```python
from build123d import *

# Parameters (mm, degrees)
BOSS_EXTRUDE1_DEPTH = 80
SHELL1_T            = -3
SKETCH3_W           = 46
SKETCH3_H           = 47
BOSS_EXTRUDE2_DEPTH = 17
SKETCH4_W           = 10.2
SKETCH4_H           = 10.2
CUT_EXTRUDE1_DEPTH  = 20
SKETCH6_W           = 15
SKETCH6_H           = 12.8
CUT_EXTRUDE2_DEPTH  = 3
SKETCH7_W           = 40.4
SKETCH7_H           = 50
CUT_EXTRUDE3_DEPTH  = 5
FILLET1_R           = 4
CUT_EXTRUDE7_DEPTH  = 47
SKETCH13_R          = 1.5
CUT_EXTRUDE8_DEPTH  = 25
SKETCH14_R          = 3.1
CUT_EXTRUDE9_DEPTH  = 2
SKETCH17_W          = 45
SKETCH17_H          = 5
BOSS_EXTRUDE5_DEPTH = 74
CUT_EXTRUDE10_REACH = 48.51
SKETCH18_W          = 54
SKETCH18_H          = 45
CUT_EXTRUDE11_REACH = 48.51
SKETCH19_R          = 1.45
BOSS_EXTRUDE6_DEPTH = 47
SKETCH22_R          = 1.45
CUT_EXTRUDE12_DEPTH = 70.509632224
CUT_EXTRUDE13_REACH = 82
SKETCH24_R          = 3.7
SKETCH24_W          = 2
SKETCH24_H          = 3
BOSS_EXTRUDE7_DEPTH = 74
SKETCH27_R          = 1.65
CUT_EXTRUDE14_DEPTH = 10
CUT_EXTRUDE15_START = -3
CUT_EXTRUDE15_DEPTH = 32
CUT_EXTRUDE16_DEPTH = 30
BOSS_EXTRUDE8_DEPTH = 20
SKETCH31_R          = 1.5
CUT_EXTRUDE17_DEPTH = 43.509632224
CUT_EXTRUDE18_DEPTH = 15
CUT_EXTRUDE19_REACH = 48.51
SKETCH33_W          = 10
SKETCH33_H          = 5
SKETCH34_R          = 1.6
CUT_EXTRUDE20_DEPTH = 70.509632224
CUT_EXTRUDE22_DEPTH = 14


with BuildPart() as part:
    # Sketch2 → Boss-Extrude1 (new body)
    with BuildSketch(Plane(origin=(0, 0, 0), x_dir=(0, 0, -1), z_dir=(1, 0, 0))):
        Polygon((-27.320490368, 20.998248687), (-27.320490368, -29.001751313), (12.679509632, -29.001751313), (12.679509632, -48.511383538), (27.679509632, -48.511383538), (82.679509632, 0.998248687), (82.679509632, 20.998248687), align=None)
    extrude(amount=BOSS_EXTRUDE1_DEPTH)

    # Shell1
    shell1_openings = [part.faces().sort_by_distance(p)[0] for p in [
        (40, 20.998248687, -27.679509632),
    ]]
    offset(amount=SHELL1_T, openings=shell1_openings, kind=Kind.INTERSECTION)

    # Sketch3 → Boss-Extrude2 (add)
    with BuildSketch(Plane(origin=(0, 0, 24.320490368), x_dir=(-1, 0, 0), z_dir=(0, 0, -1))):
        with Locations((-40, -2.501751313)):
            Rectangle(SKETCH3_W, SKETCH3_H)
    extrude(amount=BOSS_EXTRUDE2_DEPTH)

    # Sketch4 → Cut-Extrude1 (cut)
    with BuildSketch(Plane.XY.offset(27.320490368)):
        with Locations((40, -4.001751313)):
            Rectangle(SKETCH4_W, SKETCH4_H)
    extrude(amount=-CUT_EXTRUDE1_DEPTH, mode=Mode.SUBTRACT)

    # Sketch6 → Cut-Extrude2 (cut)
    with BuildSketch(Plane.XZ.offset(29.001751313)):
        with Locations((51.5, 0.920490368)):
            Rectangle(SKETCH6_W, SKETCH6_H)
        with Locations((28.5, 0.920490368)):
            Rectangle(SKETCH6_W, SKETCH6_H)
    extrude(amount=-CUT_EXTRUDE2_DEPTH, mode=Mode.SUBTRACT)

    # Sketch7 → Cut-Extrude3 (cut)
    with BuildSketch(Plane.XY.offset(27.320490368)):
        with Locations((40, -4.001751313)):
            Rectangle(SKETCH7_W, SKETCH7_H)
    extrude(amount=-CUT_EXTRUDE3_DEPTH, mode=Mode.SUBTRACT)

    # Fillet1
    fillet1_edges = [part.edges().sort_by_distance(p)[0] for p in [
        (19.8, -4.001751313, 27.320490368),
        (60.2, -4.001751313, 27.320490368),
        (80, -4.001751313, 27.320490368),
        (0, -4.001751313, 27.320490368),
    ]]
    fillet(fillet1_edges, radius=FILLET1_R)

    # Sketch12 → Cut-Extrude7 (cut)
    with BuildSketch(Plane(origin=(0, 20.998248687, 0), x_dir=(1, 0, 0), z_dir=(0, 1, 0))):
        Polygon((33, -7.320490368), (19.8, -12.320490368), (17, -24.320490368), (17, -7.320490368), align=None)
        Polygon((47, -7.320490368), (63, -7.320490368), (63, -24.320490368), (60.2, -12.320490368), align=None)
    extrude(amount=-CUT_EXTRUDE7_DEPTH, mode=Mode.SUBTRACT)

    # Sketch13 → Cut-Extrude8 (cut)
    with BuildSketch(Plane(origin=(0, 20.998248687, 0), x_dir=(1, 0, 0), z_dir=(0, 1, 0))):
        with Locations((26, -17.320490368)):
            Circle(SKETCH13_R)
        with Locations((54, -17.320490368)):
            Circle(SKETCH13_R)
    extrude(amount=-CUT_EXTRUDE8_DEPTH, mode=Mode.SUBTRACT)

    # Sketch14 → Cut-Extrude9 (cut)
    with BuildSketch(Plane(origin=(0, 20.998248687, 0), x_dir=(1, 0, 0), z_dir=(0, 1, 0))):
        with Locations((26, -17.320490368)):
            Circle(SKETCH14_R)
        with Locations((54, -17.320490368)):
            Circle(SKETCH14_R)
    extrude(amount=-CUT_EXTRUDE9_DEPTH, mode=Mode.SUBTRACT)

    # Sketch17 → Boss-Extrude5 (add)
    with BuildSketch(Plane.ZY.offset(-77)):
        with Locations((-23.179509632, -4.501751313)):
            Rectangle(SKETCH17_W, SKETCH17_H)
    extrude(amount=BOSS_EXTRUDE5_DEPTH)

    # Sketch18 → Cut-Extrude10 (cut, up to next)
    with BuildSketch(Plane(origin=(0, -2.001751313, 0), x_dir=(1, 0, 0), z_dir=(0, 1, 0)), mode=Mode.PRIVATE) as cut_extrude10_sk1:
        with Locations((40, 23.179509632)):
            Rectangle(SKETCH18_W, SKETCH18_H)
    cut_extrude10_tool1 = extrude(cut_extrude10_sk1.sketch, amount=-CUT_EXTRUDE10_REACH, mode=Mode.PRIVATE) & part.part
    add(cut_extrude10_tool1.solids().sort_by_distance((40, -2.001751, -23.17951))[0], mode=Mode.SUBTRACT)

    # Sketch19 → Cut-Extrude11 (cut, up to next)
    with BuildSketch(Plane(origin=(0, -2.001751313, 0), x_dir=(1, 0, 0), z_dir=(0, 1, 0)), mode=Mode.PRIVATE) as cut_extrude11_sk1:
        with Locations((72, 37.179509632)):
            Circle(SKETCH19_R)
    cut_extrude11_tool1 = extrude(cut_extrude11_sk1.sketch, amount=-CUT_EXTRUDE11_REACH, mode=Mode.PRIVATE) & part.part
    add(cut_extrude11_tool1.solids().sort_by_distance((72, -2.001751, -37.17951))[0], mode=Mode.SUBTRACT)
    # Sketch19 → Cut-Extrude11 (cut, up to next)
    with BuildSketch(Plane(origin=(0, -2.001751313, 0), x_dir=(1, 0, 0), z_dir=(0, 1, 0)), mode=Mode.PRIVATE) as cut_extrude11_sk2:
        with Locations((72, 6.179509632)):
            Circle(SKETCH19_R)
    cut_extrude11_tool2 = extrude(cut_extrude11_sk2.sketch, amount=-CUT_EXTRUDE11_REACH, mode=Mode.PRIVATE) & part.part
    add(cut_extrude11_tool2.solids().sort_by_distance((72, -2.001751, -6.17951))[0], mode=Mode.SUBTRACT)
    # Sketch19 → Cut-Extrude11 (cut, up to next)
    with BuildSketch(Plane(origin=(0, -2.001751313, 0), x_dir=(1, 0, 0), z_dir=(0, 1, 0)), mode=Mode.PRIVATE) as cut_extrude11_sk3:
        with Locations((8, 33.179509632)):
            Circle(SKETCH19_R)
    cut_extrude11_tool3 = extrude(cut_extrude11_sk3.sketch, amount=-CUT_EXTRUDE11_REACH, mode=Mode.PRIVATE) & part.part
    add(cut_extrude11_tool3.solids().sort_by_distance((8, -2.001751, -33.17951))[0], mode=Mode.SUBTRACT)
    # Sketch19 → Cut-Extrude11 (cut, up to next)
    with BuildSketch(Plane(origin=(0, -2.001751313, 0), x_dir=(1, 0, 0), z_dir=(0, 1, 0)), mode=Mode.PRIVATE) as cut_extrude11_sk4:
        with Locations((8, 6.179509632)):
            Circle(SKETCH19_R)
    cut_extrude11_tool4 = extrude(cut_extrude11_sk4.sketch, amount=-CUT_EXTRUDE11_REACH, mode=Mode.PRIVATE) & part.part
    add(cut_extrude11_tool4.solids().sort_by_distance((8, -2.001751, -6.17951))[0], mode=Mode.SUBTRACT)

    # Sketch21 → Boss-Extrude6 (add)
    with BuildSketch(Plane(origin=(0, -26.001751313, 0), x_dir=(1, 0, 0), z_dir=(0, 1, 0))):
        Polygon((3, -24.320490368), (3, -14.320490368), (19.333333333, -14.320490368), (17, -24.320490368), align=None)
    extrude(amount=BOSS_EXTRUDE6_DEPTH)

    # Sketch22 → Cut-Extrude12 (cut, through all)
    with BuildSketch(Plane(origin=(0, 20.998248687, 0), x_dir=(1, 0, 0), z_dir=(0, 1, 0))):
        with Locations((10, -19.320490368)):
            Circle(SKETCH22_R)
    extrude(amount=-CUT_EXTRUDE12_DEPTH, mode=Mode.SUBTRACT)

    # Sketch24 → Cut-Extrude13 (cut, up to next)
    with BuildSketch(Plane(origin=(80, 0, 0), x_dir=(0, 0, -1), z_dir=(1, 0, 0)), mode=Mode.PRIVATE) as cut_extrude13_sk1:
        with Locations((26.679509632, -30.511383538)):
            Circle(SKETCH24_R)
    cut_extrude13_tool1 = extrude(cut_extrude13_sk1.sketch, amount=-CUT_EXTRUDE13_REACH, mode=Mode.PRIVATE) & part.part
    add(cut_extrude13_tool1.solids().sort_by_distance((80, -30.511384, -26.67951))[0], mode=Mode.SUBTRACT)
    # Sketch24 → Cut-Extrude13 (cut, up to next)
    with BuildSketch(Plane(origin=(80, 0, 0), x_dir=(0, 0, -1), z_dir=(1, 0, 0)), mode=Mode.PRIVATE) as cut_extrude13_sk2:
        with Locations((34.379509632, -30.511383538)):
            Rectangle(SKETCH24_W, SKETCH24_H)
    cut_extrude13_tool2 = extrude(cut_extrude13_sk2.sketch, amount=-CUT_EXTRUDE13_REACH, mode=Mode.PRIVATE) & part.part
    add(cut_extrude13_tool2.solids().sort_by_distance((80, -30.511384, -34.37951))[0], mode=Mode.SUBTRACT)

    # Sketch26 → Boss-Extrude7 (add)
    with BuildSketch(Plane(origin=(3, 0, 0), x_dir=(0, 0, -1), z_dir=(1, 0, 0))):
        Polygon((79.679509632, 2.334161996), (63.679509632, 2.334161996), (63.679509632, -12.068640106), align=None)
    extrude(amount=BOSS_EXTRUDE7_DEPTH)

    # Sketch27 → Cut-Extrude14 (cut)
    with BuildSketch(Plane(origin=(0, 2.334161996, 0), x_dir=(1, 0, 0), z_dir=(0, 1, 0))):
        with Locations((6, 76.679509632)):
            Circle(SKETCH27_R)
        with Locations((74, 76.679509632)):
            Circle(SKETCH27_R)
    extrude(amount=-CUT_EXTRUDE14_DEPTH, mode=Mode.SUBTRACT)

    # Sketch28 → Cut-Extrude15 (cut)
    with BuildSketch(Plane(origin=(0, 2.334161996, 0), x_dir=(1, 0, 0), z_dir=(0, 1, 0)).offset(CUT_EXTRUDE15_START)):
        Polygon((74, 79.929509632), (71.185417438, 78.304509632), (71.185417438, 75.054509632), (74, 73.429509632), (76.814582562, 75.054509632), (76.814582562, 78.304509632), align=None)
        Polygon((6, 73.429509632), (8.814582562, 75.054509632), (8.814582562, 78.304509632), (6, 79.929509632), (3.185417438, 78.304509632), (3.185417438, 75.054509632), align=None)
    extrude(amount=-CUT_EXTRUDE15_DEPTH, mode=Mode.SUBTRACT)

    # Sketch29 → Cut-Extrude16 (cut)
    with BuildSketch(Plane.XZ.offset(29.001751313)):
        Polygon((7.185417438, 17.695490368), (10, 16.070490368), (12.814582562, 17.695490368), (12.814582562, 20.945490368), (10, 22.570490368), (7.185417438, 20.945490368), align=None)
    extrude(amount=-CUT_EXTRUDE16_DEPTH, mode=Mode.SUBTRACT)

    # Sketch30 → Boss-Extrude8 (add)
    with BuildSketch(Plane(origin=(0, -26.001751313, 0), x_dir=(1, 0, 0), z_dir=(0, 1, 0))):
        Polygon((77, -24.320490368), (63, -24.320490368), (60.2, -12.320490368), (77, -12.320490368), align=None)
    extrude(amount=BOSS_EXTRUDE8_DEPTH)

    # Sketch31 → Cut-Extrude17 (cut, through all)
    with BuildSketch(Plane(origin=(0, -6.001751313, 0), x_dir=(1, 0, 0), z_dir=(0, 1, 0))):
        with Locations((72, -21.320490368)):
            Circle(SKETCH31_R)
    extrude(amount=-CUT_EXTRUDE17_DEPTH, mode=Mode.SUBTRACT)

    # Sketch32 → Cut-Extrude18 (cut)
    with BuildSketch(Plane.XZ.offset(29.001751313)):
        Polygon((72, 24.570490368), (69.185417438, 22.945490368), (69.185417438, 19.695490368), (72, 18.070490368), (74.814582562, 19.695490368), (74.814582562, 22.945490368), align=None)
    extrude(amount=-CUT_EXTRUDE18_DEPTH, mode=Mode.SUBTRACT)

    # Sketch33 → Cut-Extrude19 (cut, up to next)
    with BuildSketch(Plane(origin=(0, -2.001751313, 0), x_dir=(1, 0, 0), z_dir=(0, 1, 0)), mode=Mode.PRIVATE) as cut_extrude19_sk1:
        with Locations((72, 43.179509632)):
            Rectangle(SKETCH33_W, SKETCH33_H)
    cut_extrude19_tool1 = extrude(cut_extrude19_sk1.sketch, amount=-CUT_EXTRUDE19_REACH, mode=Mode.PRIVATE) & part.part
    add(cut_extrude19_tool1.solids().sort_by_distance((72, -2.001751, -43.17951))[0], mode=Mode.SUBTRACT)

    # Sketch34 → Cut-Extrude20 (cut, through all)
    with BuildSketch(Plane(origin=(0, 20.998248687, 0), x_dir=(1, 0, 0), z_dir=(0, 1, 0))):
        with Locations((40, -17.320490368)):
            Circle(SKETCH34_R)
    extrude(amount=-CUT_EXTRUDE20_DEPTH, mode=Mode.SUBTRACT)

    # Sketch36 → Cut-Extrude22 (cut)
    with BuildSketch(Plane.XZ.offset(29.001751313)):
        Polygon((38.375, 20.13507293), (36.75, 17.320490368), (38.375, 14.505907805), (41.625, 14.505907805), (43.25, 17.320490368), (41.625, 20.13507293), align=None)
    extrude(amount=-CUT_EXTRUDE22_DEPTH, mode=Mode.SUBTRACT)


solid = part.part
```
Can you work these out from the model? Positions are in its coordinate system, mm. A direction names the side the tool comes from. Coordinates: 2 decimals unless noted, no trailing zeros. Loops run counter-clockwise (first coordinate to the right, second up) from the corner with the lowest first, then second, coordinate; pieces in that order, holes last. Notation, with made-up numbers: (57.5, 36.25) -> (79.5, 36.25) arc R28 cw to (79.5, 64.25) -> close; hole circle Ø1 at (13, 68). An arc over 180 degrees is marked (long way). Answer as a JSON object with one key per item and string values.
1) Imagine slicing it at C-C (x = 17.5). Please give me the cut outline in (y, z), then the cut area to 3 significant figures.
Results:
{"outline": "(-48.51, -27.68) -> (1, -82.68) -> (21, -82.68) -> (21, -79.68) -> (2.33, -79.68) -> (2.33, -63.68) -> (-12.07, -63.68) -> (-45.51, -26.53) -> (-45.51, -15.68) -> (-26, -15.68) -> (-26, 14.32) -> (21, 14.32) -> (21, 26.94) -> (-29, 26.94) -> (-29, -12.68) -> (-48.51, -12.68) -> close", "area": "1,210 mm^2"}
2) For faces 4 (the face through (73.388, -21.607, 18.872)), 5 (the face through (39, 12, -79.68)), 6 (the face through (36, -28, 1)), 7 (the face through (61.403, -3.652, 26.18)), 8 (the face through (78.521, -30.349, -22.983)), which set-ups out of +Z, -Z, +X, -X, +Y, -Y let a thin tool reach every point of the face, with its end or its side?
Results:
{"face 4": "-Y", "face 5": "+Y", "face 6": "+Y, -Y", "face 7": "+Z, +Y, -Y", "face 8": "+X"}
3) Thinking about a two-plate mould opening in X: for faces 1 (the face through (0, -6, -29)), 2 (the face through (7.185, -14, 19)), 3 (the face through (39, -48.511, -20)), which applies, pulls with the +X half, pulls with the -X half, needs draft (parallel to the pull), parting line crosses it, or undercut?
Results:
{"face 1": "pulls with the -X half", "face 2": "undercut", "face 3": "needs draft"}
4) Imagine slicing it at D-D (y = -23). Count the separate pieces of the cut face and the enclosed holes in it, then the cut area to 3 significant figures.
Results:
{"separate pieces": "1", "enclosed holes": "4", "area": "1,750 mm^2"}
5) If I drill on line 1 (Z direction, x = 74, y = 1); line 2 (X direction, y = -28, z = -0.5); line 3 (Z direction, x = 54, y = 20.5), over which ranges is the centre line in solid material (lowest first)?
Results:
{"line 1": "z = -82.68 to -78.33, -75.03 to -63.68, 24.32 to 27.32", "line 2": "x = 0 to 21, 36 to 44, 59 to 80", "line 3": "z = -82.68 to -79.68, 9.97 to 14.22, 20.42 to 22.32"}
6) For P1, Ø1, axis at x = 36.5, z = 1, coming from the -Y side; P2, Ø2.5, axis at x = 31, y = -27, coming from the +Z side; P3, Ø2.5, axis at x = 8, z = -33.18, coming from the -Y side, each with a flat end and sliding along its axis, tell me the tip position at first contact or that it passes through.
Results:
{"P1": "stops at y = -29", "P2": "stops at z = 22.32", "P3": "stops at y = -44.69"}
7) Imagine slicing it at A-A (y = 6.5). Please give me the cut outline in (x, z), then the cut area to 3 significant figures.
Results:
{"outline": "(0, -82.68) -> (80, -82.68) -> (80, 23.32) arc R4 ccw to (76, 27.32) -> (64.2, 27.32) arc R4 ccw to (60.2, 23.32) -> (60.2, 22.32) -> (19.8, 22.32) -> (19.8, 23.32) arc R4 ccw to (15.8, 27.32) -> (4, 27.32) arc R4 ccw to (0, 23.32) -> close; hole (3, -79.68) -> (77, -79.68) -> (77, 24.32) -> (63, 24.32) -> (60.2, 12.32) -> (47, 7.32) -> (33, 7.32) -> (19.8, 12.32) -> (19.33, 14.32) -> (3, 14.32) -> close; hole circle Ø2.9 at (10, 19.32); hole circle Ø3 at (26, 17.32); hole circle Ø3.2 at (40, 17.32); hole circle Ø3 at (54, 17.32)", "area": "1,670 mm^2"}
8) Imagine slicing it at B-B (x = 54). Please give me the cut outline in (y, z), then the cut area to 3 significant figures.
Results:
{"outline": "(-48.51, -27.68) -> (1, -82.68) -> (21, -82.68) -> (21, -79.68) -> (2.33, -79.68) -> (2.33, -63.68) -> (-12.07, -63.68) -> (-45.51, -26.53) -> (-45.51, -15.68) -> (-26, -15.68) -> (-26, -5.48) -> (-29, -5.48) -> (-29, -12.68) -> (-48.51, -12.68) -> close; (-29, 7.32) -> (-26, 7.32) -> (-26, 9.97) -> (21, 9.97) -> (21, 14.22) -> (19, 14.22) -> (19, 15.82) -> (-4, 15.82) -> (-4, 18.82) -> (19, 18.82) -> (19, 20.42) -> (21, 20.42) -> (21, 22.32) -> (-29, 22.32) -> close", "area": "1,060 mm^2"}
